Geometry check sheet. Reference: the model listing, model coordinates, mm. Face numbers are marked on the shaded views. A direction names the side the tool comes from. Give positions to 0.01 mm unless a question says otherwise; leave off trailing zeros. Write each loop counter-clockwise with the first axis right and the second up, starting at its lowest first coordinate (ties: lowest second). Pieces come first, ordered by that corner, then holes. Notation, with made-up numbers: (55.25, 0.5) -> (87.25, 0.5) arc R29 cw to (87.25, 25.5) -> close; hole circle Ø6 at (-10, 40). An arc over 180 degrees is marked (long way). One line per item, written item: value.
from build123d import *

# Parameters (mm, degrees)
SKETCH1_W           = 25.6
SKETCH1_H           = 7.6
BOSS_EXTRUDE1_DEPTH = 61.2
FILLET1_R           = 2
SKETCH2_W           = 30
SKETCH2_H           = 13
BOSS_EXTRUDE2_DEPTH = 2
FILLET2_R           = 2
CUT_EXTRUDE1_DEPTH  = 25.6


with BuildPart() as part:
    # Sketch1 → Boss-Extrude1 (new body)
    with BuildSketch(Plane.XY):
        Rectangle(SKETCH1_W, SKETCH1_H)
    extrude(amount=BOSS_EXTRUDE1_DEPTH)

    # Fillet1
    fillet1_edges = [part.edges().sort_by_distance(p)[0] for p in [
        (12.8, -3.8, 30.6),
        (-12.8, -3.8, 30.6),
        (-12.8, 3.8, 30.6),
        (12.8, 3.8, 30.6),
    ]]
    fillet(fillet1_edges, radius=FILLET1_R)

    # Sketch2 → Boss-Extrude2 (add)
    with BuildSketch(Plane(origin=(0, 0, 0), x_dir=(-1, 0, 0), z_dir=(0, 0, -1))):
        Rectangle(SKETCH2_W, SKETCH2_H)
    extrude(amount=BOSS_EXTRUDE2_DEPTH)

    # Fillet2
    fillet2_edges = [part.edges().sort_by_distance(p)[0] for p in [
        (-15, -6.5, -1),
        (-15, 6.5, -1),
        (15, 6.5, -1),
        (15, -6.5, -1),
    ]]
    fillet(fillet2_edges, radius=FILLET2_R)

    # Sketch3 → Cut-Extrude1 (cut)
    with BuildSketch(Plane.ZY.offset(12.8)):
        Polygon((48.8, -1.8), (56.8, -1.8), (53.2, 1.8), (61.2, 1.8), (61.2, 3.8), (48.8, 3.8), align=None)
    extrude(amount=-CUT_EXTRUDE1_DEPTH, mode=Mode.SUBTRACT)


solid = part.part
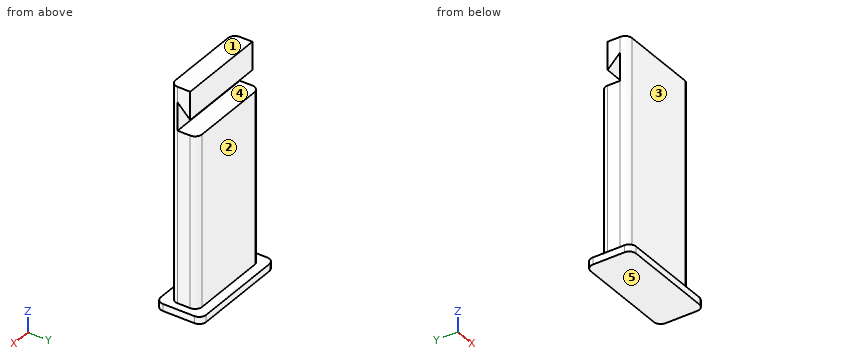
1) Sectioned sample at D-D on y = 5.25. Record the cut outline in (x, z).
Verdict:
outline: (-14.85, -2) -> (14.85, -2) -> (14.85, 0) -> (-14.85, 0) -> close
2) Sectioned sample at B-B on z = 22. Record the cut outline in (x, y), plus the area to 3 significant figures.
Verdict:
outline: (-12.8, -1.8) arc R2 ccw to (-10.8, -3.8) -> (10.8, -3.8) arc R2 ccw to (12.8, -1.8) -> (12.8, 1.8) arc R2 ccw to (10.8, 3.8) -> (-10.8, 3.8) arc R2 ccw to (-12.8, 1.8) -> close
area: 191 mm^2
3) Sectioned sample at A-A on y = -1. Record the cut outline in (x, z), plus the area to 3 significant figures.
Verdict:
outline: (-15, -2) -> (15, -2) -> (15, 0) -> (12.8, 0) -> (12.8, 48.8) -> (-12.8, 48.8) -> (-12.8, 0) -> (-15, 0) -> close; (-12.8, 56) -> (12.8, 56) -> (12.8, 61.2) -> (-12.8, 61.2) -> close
area: 1,440 mm^2
4) Mould release check, pull along Z, two halves, no side actions. Record for the marked faces 3, 4 and 5: released by +Z, released by -Z, zero draft, split by the parting line, or undercut.
Verdict:
face 3: zero draft
face 4: undercut
face 5: released by -Z
5) Tool access check on the marked faces 1 and 2. Record the directions out of +Z, -Z, +X, -X, +Y, -Y that give a thin tool (end or side, any length) a straight path to the whole face; none if there is none.
Verdict:
face 1: +Z, +X, -X, +Y, -Y
face 2: +Z, +X, -X, +Y
6) Sectioned sample at C-C on x = -7.75. Record the cut outline in (y, z).
Verdict:
outline: (-6.5, -2) -> (6.5, -2) -> (6.5, 0) -> (3.8, 0) -> (3.8, 48.8) -> (-1.8, 48.8) -> (-1.8, 56.8) -> (1.8, 53.2) -> (1.8, 61.2) -> (-3.8, 61.2) -> (-3.8, 0) -> (-6.5, 0) -> close
7) Depth check by flat-ended pin: pin 1 Ø1.1 at (y, z) = (1, 33) entering from -X; pin 2 Ø6.5 at (x, z) = (-4.5, 54) entering from +Y; pin 3 Ø1.8 at (y, z) = (0, 56) entering from +X; pin 4 Ø5 at (x, y) = (-9, 2.5) entering from +Z. Enter the tip coordinate at first touch or a pass-through.
Verdict:
pin 1: x = -12.8
pin 2: y = 1.8
pin 3: x = 12.8
pin 4: z = 61.2
8) Scan lines: probe 1 along X at (y, z) = (-2, 38); probe 2 along Y at (x, z) = (-2.5, 19); probe 3 along Z at (x, y) = (4.5, 4.5). Record each from-to range of solid material in increasing order.
Verdict:
probe 1: -12.79 to 12.79
probe 2: -3.8 to 3.8
probe 3: -2 to 0
